Can you work these out from the drawing? Everything is in mm from the part's minimum corner. A direction names the side the tool comes from. Round coordinates to 2 decimals unless told otherwise and drop trailing zeros. Write each loop counter-clockwise with the first axis right and the second up, starting at its lowest first coordinate (ties: lowest second). Pieces come first, ordered by that corner, then holes.
Q1. Please list where these lines run through material, in increasing order: line 1 along Z through (x, y) = (9.65, 3.15); line 2 along Y through (x, z) = (7, 0.95); line 3 along X through (y, z) = (0.45, 0.7).
Q2. For the marked faces 1, 2, 3 and 4, which set-ups out of +Z, -Z, +X, -X, +Y, -Y let a thin tool reach every point of the face, with its end or its side?
Q3. We'd pull the mould along X, two halves only. Please class the marked faces 5, 6 and 7: +X half, -X half, draft (parallel to the pull), parting line (faces both ways), or undercut.
Q4. I'm going to push flat-ended pins straight in: pin 1 Ø0.9 at (x, y) = (10, 3) entering from +Z; pin 2 Ø0.5 at (x, y) = (6, 5.5) entering from +Z; pin 3 Ø0.6 at (x, y) = (1, 4) entering from -Z. Where does each tip first touch, or does it pass through?
Q5. If we section it at A-A (x = 9.65): Please give me the cut outline in (y, z), plus the area to 3 significant figures.
Q6. If we section it at B-B (y = 3.55): Please give me the cut outline in (x, z).
Q7. If we section it at D-D (z = 1.5): Give the number of separate pieces and of enclosed holes in the cut face, plus the area to 3 significant figures.
Q8. If we section it at C-C (x = 1.1): Please give me the cut outline in (y, z).
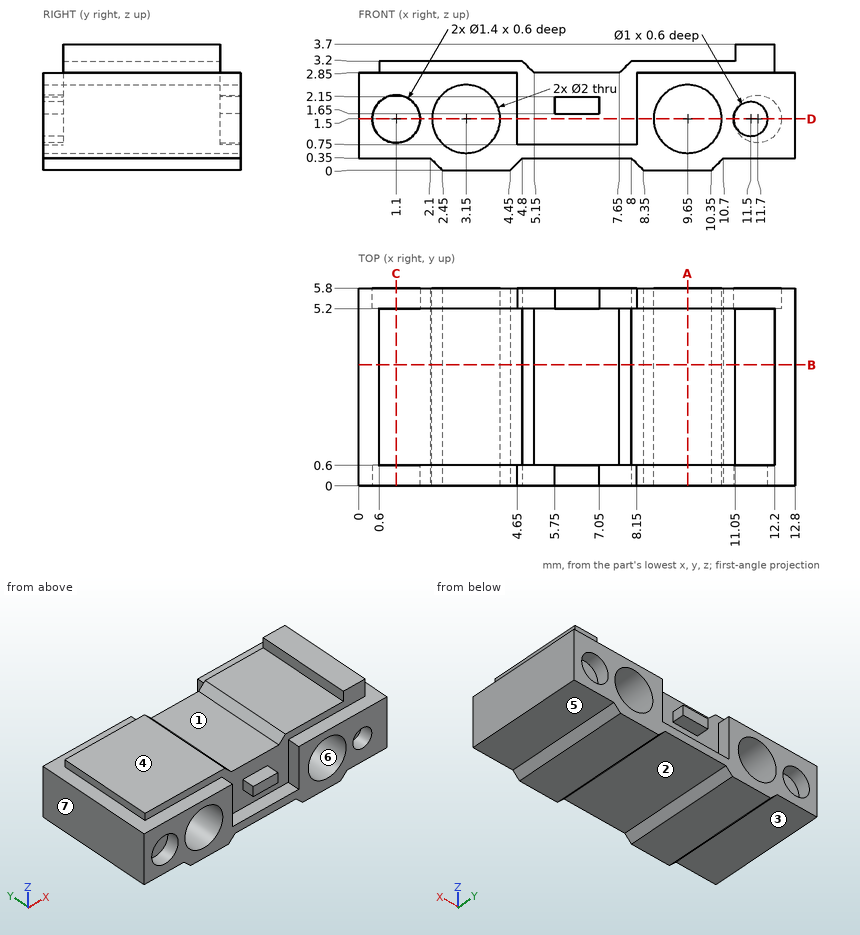
A:
1. line 1: z = 0 to 0.5, 2.5 to 3.2
1. line 2: y = 0.6 to 5.2
1. line 3: x = 0 to 2.55, 3.75 to 9.05, 10.25 to 12.8
2. face 1: +Z, +Y, -Y
2. face 2: -Z, +Y, -Y
2. face 3: -Z, -X, +Y, -Y
2. face 4: +Z, -X, +Y, -Y
3. face 5: draft
3. face 6: undercut
3. face 7: -X half
4. pin 1: stops at z = 3.2
4. pin 2: stops at z = 2.15
4. pin 3: stops at z = 0.35
5. outline: (0, 0) - (5.8, 0) - (5.8, 0.5) - (0, 0.5) - close; (0, 2.5) - (5.8, 2.5) - (5.8, 2.85) - (5.2, 2.85) - (5.2, 3.2) - (0.6, 3.2) - (0.6, 2.85) - (0, 2.85) - close
5. area: 6.54 mm2
6. outline: (0, 0.35) - (2.1, 0.35) - (2.45, 0) - (4.45, 0) - (4.8, 0.35) - (8, 0.35) - (8.35, 0) - (10.35, 0) - (10.7, 0.35) - (12.8, 0.35) - (12.8, 2.85) - (12.2, 2.85) - (12.2, 3.7) - (11.05, 3.7) - (11.05, 3.2) - (8, 3.2) - (7.65, 2.85) - (5.15, 2.85) - (4.8, 3.2) - (0.6, 3.2) - (0.6, 2.85) - (0, 2.85) - close; hole circle Ø2 at (3.15, 1.5); hole circle Ø2 at (9.65, 1.5)
7. separate pieces: 3
7. enclosed holes: 0
7. area: 43.7 mm2
8. outline: (0, 0.35) - (5.8, 0.35) - (5.8, 0.8) - (5.2, 0.8) - (5.2, 2.2) - (5.8, 2.2) - (5.8, 2.85) - (5.2, 2.85) - (5.2, 3.2) - (0.6, 3.2) - (0.6, 2.85) - (0, 2.85) - (0, 2.2) - (0.6, 2.2) - (0.6, 0.8) - (0, 0.8) - close
